For this review, take the finished solid that the model builds, in its own axes (mm). A direction names the side the tool comes from. Round coordinates to 2 decimals unless told otherwise and drop trailing zeros. Loops run counter-clockwise (first coordinate to the right, second up) from the corner with the lowest first, then second, coordinate; pieces in that order, holes last.
1. Tool access review of faces 3 (the cylindrical face through (-0.96, 0.74, -39.81)), 4 (the cylindrical face through (-23.74, 3.23, -28.65)): name each direction out of +Z, -Z, +X, -X, +Y, -Y from which nothing blocks a thin tool from reaching the whole face with its end or side.
2. Consider section D-D on z = -32. State the section outline as (x, y) points, then the cut area to 3 significant figures.
3. Consider section A-A on x = 38.5. State the section outline as (y, z) points.
4. Clearance check with flat-ended pins moving along their axes: pin 1 Ø5.5 at (x, z) = (-0.5, -38) entering from +Y; pin 2 Ø1 at (x, y) = (-10.5, 1) entering from -Z; pin 3 Ø1 at (x, y) = (-14, 3.5) entering from -Z. State where each tip first meets the part, or that it passes through.
5. Consider section C-C on y = 2.85. State how many separate pieces and enclosed holes the cut face has, then the cut area to 3 significant figures.
6. To check wall thickness, follow line 1 along Z through (x, y) = (-28, 4.1); line 2 along Z through (x, y) = (29.5, 1.85); line 3 along Z through (x, y) = (1.5, 1.35) (3 decimals). State the ranges of each line that lie inside material, in increasing order.
7. Consider section B-B on z = 37.5. State the section outline as (x, y) points, then the cut area to 3 significant figures.
8. Draft analysis for pull direction Z (two halves, no side actions). For faces 1 (the cylindrical face through (0, 3, -34)), 2 (the flat face through (1, 0, -9)), state which applies: released by +Z, released by -Z, zero draft, split by the parting line, or undercut.
Autodesk Inventor part; units mm, degrees
ref_plane "YZ Plane" through (0, 0, 0) normal (1, 0, 0) x (0, 1, 0)
ref_plane "XZ Plane" through (0, 0, 0) normal (0, 1, 0) x (-1, 0, 0)
ref_plane "XY Plane" through (0, 0, 0) normal (0, 0, 1) x (1, 0, 0)
sketch "Sketch1" plane through (0, 0, 0) normal (0, 1, 0) x (-1, 0, 0)
  circle A0 centre (0, 0) radius 45
  dimension "d0" = 90
extrude "Extrusion1" add sketch "Sketch1" along normal blind 5
sketch "Sketch2" plane through (0, 5, 0) normal (0, 1, 0) x (1, 0, 0)
  point P0 (0, 0)
  point P1 (0, -37.5)
  dimension "d17" = 37.5
sketch "Sketch3" plane through (0, 5, 0) normal (0, 1, 0) x (1, 0, 0)
  circle A0 centre (0, -22.5) radius 4.1
  circle A1 centre (0, 22.5) radius 4.1
  line L0 (-27.2764, 0) -> (27.2764, 0) construction
  circle A2 centre (0, 0) radius 4.1
  dimension "d12" = 8.2
  dimension "d14" = 45
extrude "Extrusion3" cut sketch "Sketch3" against normal up to surface (5 mm away)
hole "Hole1" at (0, 5, 37.5) direction (0, -1, 0) diameter 5 end through all counterbore diameter 7 counterbore depth 3.5
pattern_circular "Circular Pattern2" count 8 over 360 about axis through (0, 0, 0) along (0, 1, 0) of "Hole1"
Resolved:
1. face 3: +Y, -Y
1. face 4: +Y
2. outline: (-31.64, 0) - (31.64, 0) - (31.64, 5) - (-31.64, 5) - close
2. area: 316 mm2
3. outline: (0, -23.3) - (5, -23.3) - (5, -3.35) - (1.5, -3.35) - (1.5, -2.29) - (0, -2.29) - close; (0, 2.29) - (1.5, 2.29) - (1.5, 3.35) - (5, 3.35) - (5, 23.3) - (0, 23.3) - close
4. pin 1: stops at y = 1.5
4. pin 2: stops at z = -43.87
4. pin 3: stops at z = -42.93
5. separate pieces: 1
5. enclosed holes: 11
5. area: 5,900 mm2
6. line 1: z = -35.23 to -29.69, -23.35 to 23.35, 29.69 to 35.23
6. line 2: z = -33.98 to -28.35, -24.69 to 24.69, 28.35 to 33.98
6. line 3: z = -44.975 to -39.5, -35.5 to -26.316, -18.684 to -3.816, 3.816 to 18.684, 26.316 to 35.5, 39.5 to 44.975
7. outline: (-24.87, 0) - (-2.5, 0) - (-2.5, 1.5) - (-3.5, 1.5) - (-3.5, 5) - (-24.87, 5) - close; (2.5, 0) - (24.87, 0) - (24.87, 5) - (3.5, 5) - (3.5, 1.5) - (2.5, 1.5) - close
7. area: 217 mm2
8. face 1: undercut
8. face 2: zero draft
